Source: three-view drawing plus pictorial views. Frame: mm from the lowest corner of the part. Give positions to 0.01 mm unless a question says otherwise; leave off trailing zeros. Loops run counter-clockwise (first coordinate to the right, second up) from the corner with the lowest first, then second, coordinate; pieces in that order, holes last. Notation, with made-up numbers: M 2.5,74.25 L 45.5,74.25 A28 ccw 45.5,110.25 Z; hole C 7,78 d7. An arc over 180 degrees is marked long. Answer as a JSON object with one key per item and string values. Group by question number.
1) Section query C-C on z = 5. Return loops of the section in (x, y), plus the area to 3 significant figures.
2) Section query A-A on y = 6. Return loops of the section in (x, z), plus the area to 3 significant figures.
3) Section query B-B on x = 6. Return loops of the section in (y, z).
4) Draft query along Y for the marked faces 1 and 2. Return one class per face: +Y half, -Y half, draft (parallel to the pull), parting line (faces both ways), or undercut.
5) Ray query, L1, parallel to Z at x = 6, y = 0.7; L2, parallel to X at y = 2.5, z = 2.75; L3, parallel to Y at x = 10, z = 8.75. Return the intervals inside material, ascending.
6) First-contact query: P1, Ø2, axis at x = 2, z = 6, coming from the -Y side; P2, Ø1, axis at y = 10, z = 17, coming from the -X side; P3, Ø2, axis at x = 6, z = 5, coming from the +Y side. Flat tips, straight axial feed; report the tip coordinate or a pass-through.
7) Section query D-D on z = 10.5. Return loops of the section in (x, y), plus the area to 3 significant figures.
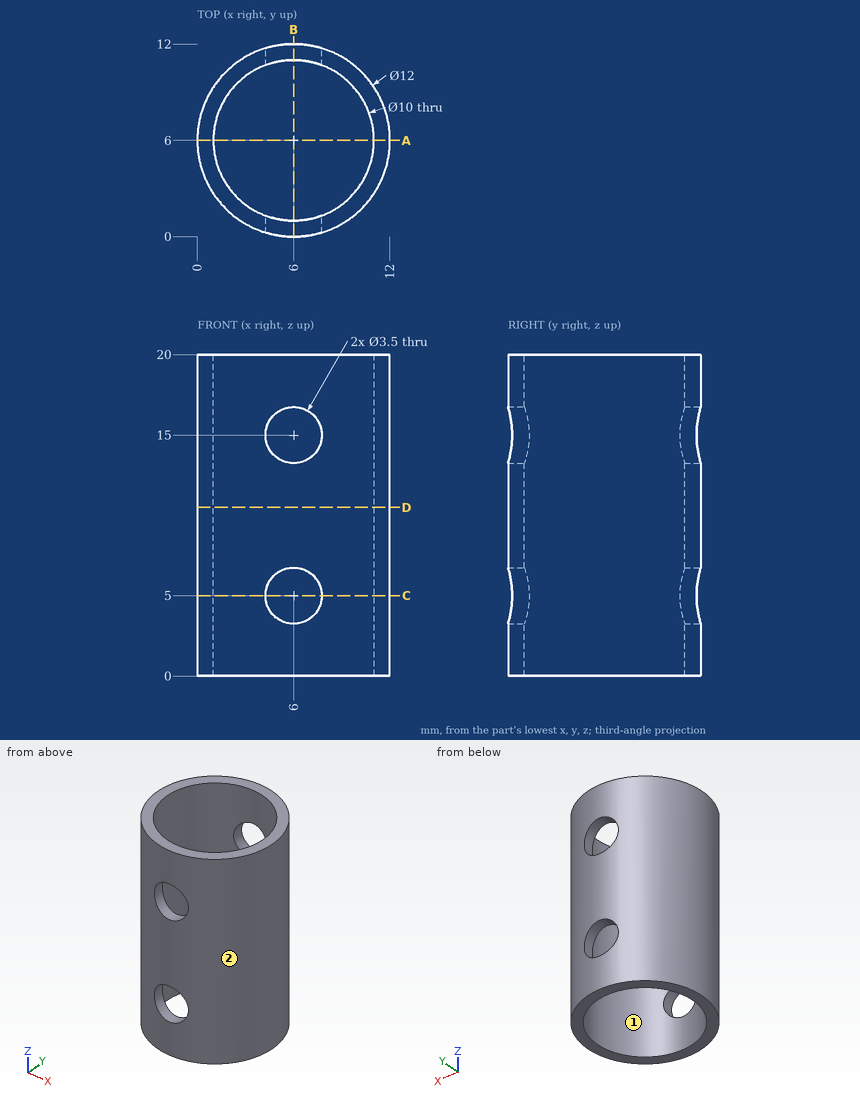
Output:
{
 "1": {"outline": "M 4.25,0.26 L 4.25,1.32 A5 cw 4.25,10.68 L 4.25,11.74 A6 ccw Z; M 7.75,0.26 A6 ccw 7.75,11.74 L 7.75,10.68 A5 cw 7.75,1.32 Z", "area": "27.4 mm^2"},
 "2": {"outline": "M 0,0 L 1,0 L 1,20 L 0,20 Z; M 11,0 L 12,0 L 12,20 L 11,20 Z", "area": "40.0 mm^2"},
 "3": {"outline": "M 0,0 L 1,0 L 1,3.25 L 0,3.25 Z; M 0,6.75 L 1,6.75 L 1,13.25 L 0,13.25 Z; M 0,16.75 L 1,16.75 L 1,20 L 0,20 Z; M 11,0 L 12,0 L 12,3.25 L 11,3.25 Z; M 11,6.75 L 12,6.75 L 12,13.25 L 11,13.25 Z; M 11,16.75 L 12,16.75 L 12,20 L 11,20 Z"},
 "4": {"face 1": "undercut", "face 2": "parting line"},
 "5": {"L1": "z = 0 to 3.25, 6.75 to 13.25, 16.75 to 20", "L2": "x = 1.13 to 2.43, 9.57 to 10.87", "L3": "y = 1.53 to 3, 9 to 10.47"},
 "6": {"P1": "stops at y = 0.8", "P2": "stops at x = 1.13", "P3": "passes through"},
 "7": {"outline": "C 6,6 d12; hole C 6,6 d10", "area": "34.6 mm^2"}
}
